from build123d import *

# Parameters (mm, degrees)
F2_R    = 1.27
F3_SIZE = 0.254


with BuildPart() as f1:
    # F0 (on Front) → F1 (revolve)
    with BuildSketch(Plane.XZ):
        with BuildLine():
            Line((-22.225, -38.1), (-22.225, 0))
            Line((-22.225, 0), (-23.8125, 0))
            ThreePointArc((-23.8125, 0), (-25.4, -1.5875), (-26.9875, 0))
            Line((-26.9875, 0), (-28.575, 0))
            Line((-28.575, 0), (-30.1625, -1.5875))
            Line((-30.1625, -1.5875), (-30.1625, -6.35))
            Line((-30.1625, -6.35), (-23.8125, -6.35))
            Line((-23.8125, -6.35), (-23.8125, -15.875))
            Line((-23.8125, -15.875), (-24.638, -15.875))
            ThreePointArc((-24.638, -15.875), (-25.176815, -16.098185), (-25.4, -16.637))
            Line((-25.4, -16.637), (-25.4, -38.1))
            Line((-25.4, -38.1), (-22.225, -38.1))
        make_face()
    revolve(axis=Axis((0, 0, -15.143116), (0, 0, -1)))

    # F2
    f2_edges = [f1.edges().sort_by_distance(p)[0] for p in [
        (23.8125, 0, -6.35),
    ]]
    fillet(f2_edges, radius=F2_R)

    # F3
    f3_edges = [f1.edges().sort_by_distance(p)[0] for p in [
        (30.1625, 0, -6.35),
        (25.4, 0, -38.1),
        (22.225, 0, 0),
        (22.225, 0, -38.1),
    ]]
    chamfer(f3_edges, length=F3_SIZE)


solid = f1.part
Read the model definition and answer for the solid it produces. Units are mm, in the model's axes. A direction names the side the tool comes from. Coordinates: 2 decimals unless noted, no trailing zeros. Loops run counter-clockwise (first coordinate to the right, second up) from the corner with the lowest first, then second, coordinate; pieces in that order, holes last.
Q1. The part is cut by section C-C on z = -29.5. Write down the section's boundary in (x, y) (3 decimals), and give its area (3 significant figures).
Q2. Each of these flat-tipped pins is pushed along its axis until it touches: pin 1 Ø1 at (x, y) = (21.5, -10.5) entering from +Z; pin 2 Ø5 at (y, z) = (-7.5, -8) entering from -X. Where does it stop, or does it pass through?
Q3. Consider probe 1 along Y at (x, z) = (0, -23) (3 decimals); probe 2 along Y at (x, z) = (0, -10) (1 decimal); probe 3 along X at (y, z) = (-10.5, -23.5). Determine where each line is inside the solid, lowest interval first.
Q4. The mould has two halves that part along X. Classify faces 3 (the face through (-21.199, 6.676, -18.787)), 4 (the face through (16, -20, -6.35)), 5 (the face through (5.506, -24.796, -27.39)): +X half, -X half, draft (parallel to the pull), parting line (faces both ways), or undercut.
Q5. Which of the six approach directions +Z, -Z, +X, -X, +Y, -Y give full straight-line access (tool end or side, diameter ignored) to faces 1 (the face through (18.897, -14.49, -11.805)), 2 (the face through (10.4, -25.3, 0))?
Results below:
1. outline: circle Ø50.8 at (0, 0); hole circle Ø44.45 at (0, 0)
1. area: 475 mm2
2. pin 1: stops at z = 0
2. pin 2: stops at x = -29.58
3. probe 1: y = -25.4 to -22.225, 22.225 to 25.4
3. probe 2: y = -23.8 to -22.2, 22.2 to 23.8
3. probe 3: x = -23.13 to -19.59, 19.59 to 23.13
4. face 3: undercut
4. face 4: draft
4. face 5: parting line
5. face 1: none
5. face 2: +Z, +X, -X, +Y, -Y
